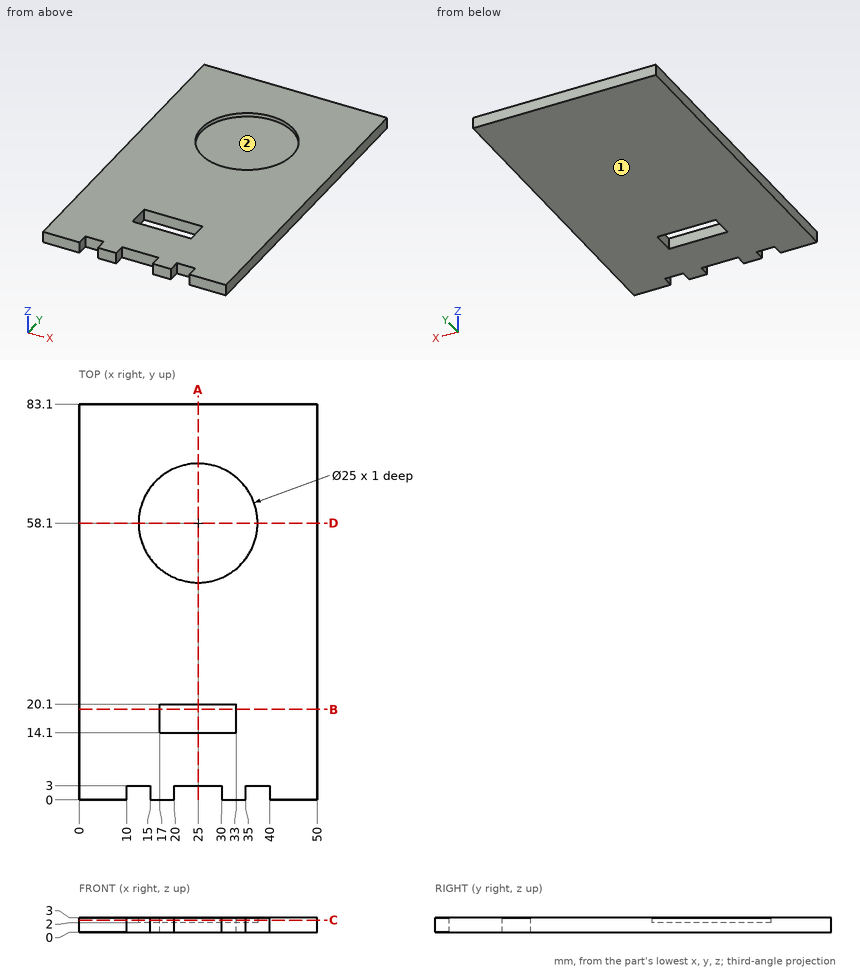
The drawing under review shows one solid part. Ordinate dimensions are in mm from its lowest x, y, z. Coordinates: 2 decimals unless noted, no trailing zeros. Write each loop counter-clockwise with the first axis right and the second up, starting at its lowest first coordinate (ties: lowest second). Pieces come first, ordered by that corner, then holes. Notation, with made-up numbers: (86.5, 73) - (129.5, 73) arc R23 cw to (129.5, 93) - close; hole circle Ø9 at (66.5, 57). An arc over 180 degrees is marked (long way). Answer in a Markdown table with one row per item. Add a question column.
Q1. We need section C-C, the plane z = 2.5. State the section outline as (x, y) points, and give its area (3 significant figures).
Q2. We need section D-D, the plane y = 58.1. State the section outline as (x, z) points.
Q3. For probe 1 along Y at (x, z) = (25, 2.5); probe 2 along Y at (x, z) = (18.5, 0.55); probe 3 along X at (y, z) = (16, 1.85), list the stretches that pass through material, from the lowest coordinate up.
Q4. We need section B-B, the plane y = 19. State the section outline as (x, z) points, and give its area (3 significant figures).
Q5. We need section A-A, the plane x = 25. State the section outline as (y, z) points.
Q6. For P1, Ø0.9, axis at x = 13, z = 1, coming from the -Y side; P2, Ø12.5, axis at x = 19.5, y = 61, coming from the +Z side, all flat-tipped, find the tip position at first contact; note any pin that passes through.
Q7. Draft analysis for pull direction X (two halves, no side actions). For the marked faces 1 and 2, state which applies: +X half, -X half, draft (parallel to the pull), parting line (faces both ways), or undercut.
Answer list:
| question | item | result |
|---|---|---|
| 1 | outline | (0, 0) - (10, 0) - (10, 3) - (15, 3) - (15, 0) - (20, 0) - (20, 3) - (30, 3) - (30, 0) - (35, 0) - (35, 3) - (40, 3) - (40, 0) - (50, 0) - (50, 83.1) - (0, 83.1) - close; hole circle Ø25 at (25, 58.1); hole (17, 14.1) - (33, 14.1) - (33, 20.1) - (17, 20.1) - close |
| 1 | area | 3,510 mm2 |
| 2 | outline | (0, 0) - (50, 0) - (50, 3) - (37.5, 3) - (37.5, 2) - (12.5, 2) - (12.5, 3) - (0, 3) - close |
| 3 | probe 1 | y = 3 to 14.1, 20.1 to 45.6, 70.6 to 83.1 |
| 3 | probe 2 | y = 0 to 14.1, 20.1 to 83.1 |
| 3 | probe 3 | x = 0 to 17, 33 to 50 |
| 4 | outline | (0, 0) - (17, 0) - (17, 3) - (0, 3) - close; (33, 0) - (50, 0) - (50, 3) - (33, 3) - close |
| 4 | area | 102 mm2 |
| 5 | outline | (3, 0) - (14.1, 0) - (14.1, 3) - (3, 3) - close; (20.1, 0) - (83.1, 0) - (83.1, 3) - (70.6, 3) - (70.6, 2) - (45.6, 2) - (45.6, 3) - (20.1, 3) - close |
| 6 | P1 | stops at y = 3 |
| 6 | P2 | stops at z = 2 |
| 7 | face 1 | draft |
| 7 | face 2 | undercut |
